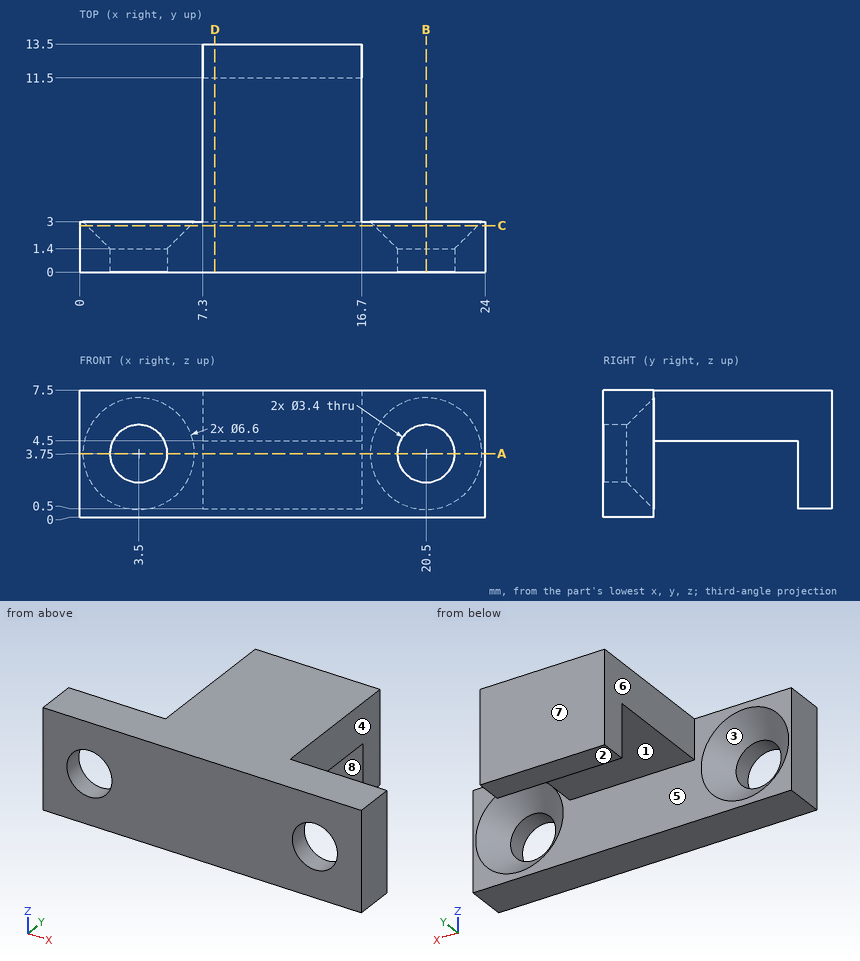
Drawing for the job (mm, zero at the part's lowest x, y, z). A direction names the side the tool comes from. Give positions to 0.01 mm unless a question says otherwise; leave off trailing zeros. Order: outer loops, then holes, each group sorted by start corner. A loop starts at its lowest first (then second) coordinate and runs counter-clockwise, first axis right, second up. Notation, with made-up numbers: M -34,36 L -28,36 A28 cw -28,67 Z; hole C 5.25,12 d9. An arc over 180 degrees is marked long. Put each result on its own line as item: value. Start each with the question number.
(1) Saw through at A-A, the plane z = 3.75. Write the cut outline in (x, y), then the cut area to 3 significant figures.
(2) Flat gauge pins, fed straight in: pin 1 Ø3.5 at (y, z) = (7, 5) entering from -X; pin 2 Ø2 at (y, z) = (7, 5.5) entering from +X; pin 3 Ø4 at (x, y) = (10.5, 6.5) entering from -Z; pin 4 Ø2 at (x, z) = (20.5, 3.75) entering from +Y. Where does each tip first touch, or does it go through?
(3) Saw through at C-C, the plane y = 2.75. Write the cut outline in (x, z).
(4) Which spindle directions (+Z, -Z, +X, -X, +Y, -Y) get a long thin tool onto all of the face, cutting with end or side? Do the marked faces 1, 2, 3, 4 and 5. Say none if no direction does.
(5) Mould opens along Y. For the marked faces 6, 7 and 8 say: +Y half, -Y half, draft (parallel to the pull), parting line (faces both ways), or undercut.
(6) Saw through at B-B, the plane x = 20.5. Write the cut outline in (y, z).
(7) Drill centre lines: line 1 along Z through (x, y) = (20.5, 0.4); line 2 along Y through (x, z) = (16, 3.75); line 3 along X through (y, z) = (1.75, 2.25). Where is each one in solid material? Low to high.
(8) Saw through at D-D, the plane x = 8. Write the cut outline in (y, z).
Check result:
1. outline: M 0,0 L 1.8,0 L 1.8,1.4 L 0.2,3 L 0,3 Z; M 5.2,0 L 18.8,0 L 18.8,1.4 L 17.2,3 L 6.8,3 L 5.2,1.4 Z; M 7.3,11.5 L 16.7,11.5 L 16.7,13.5 L 7.3,13.5 Z; M 22.2,0 L 24,0 L 24,3 L 23.8,3 L 22.2,1.4 Z
1. area: 65.3 mm2
2. pin 1: stops at x = 7.3
2. pin 2: stops at x = 16.7
2. pin 3: stops at z = 4.5
2. pin 4: passes through
3. outline: M 0,0 L 24,0 L 24,7.5 L 0,7.5 Z; hole C 3.5,3.75 d6.1; hole C 20.5,3.75 d6.1
4. face 1: -Z, +X, -X
4. face 2: -Z, +X, -X, +Y
4. face 3: +Y
4. face 4: +Z, -Z, +X, +Y
4. face 5: -Z
5. face 6: draft
5. face 7: +Y half
5. face 8: undercut
6. outline: M 0,0 L 3,0 L 3,0.45 L 1.4,2.05 L 0,2.05 Z; M 0,5.45 L 1.4,5.45 L 3,7.05 L 3,7.5 L 0,7.5 Z
7. line 1: z = 0 to 2.05, 5.45 to 7.5
7. line 2: y = 0 to 3, 11.5 to 13.5
7. line 3: x = 0 to 2.1, 4.9 to 19.1, 21.9 to 24
8. outline: M 0,0 L 3,0 L 3,4.5 L 11.5,4.5 L 11.5,0.5 L 13.5,0.5 L 13.5,7.5 L 0,7.5 Z
